The model under review builds one solid part; all positions refer to its coordinate system, in mm. Face numbers are marked on the shaded views. Give positions to 0.01 mm unless a question says otherwise; leave off trailing zeros. Order: outer loops, then holes, each group sorted by start corner. A loop starts at its lowest first (then second) coordinate and runs counter-clockwise, first axis right, second up. Notation, with made-up numbers: (82, 34.25) -> (107, 34.25) arc R12 ccw to (107, 43.25) -> close; hole circle Ø4 at (-24, 53.5). An arc over 180 degrees is marked (long way). Use one line per item in the form item = value.
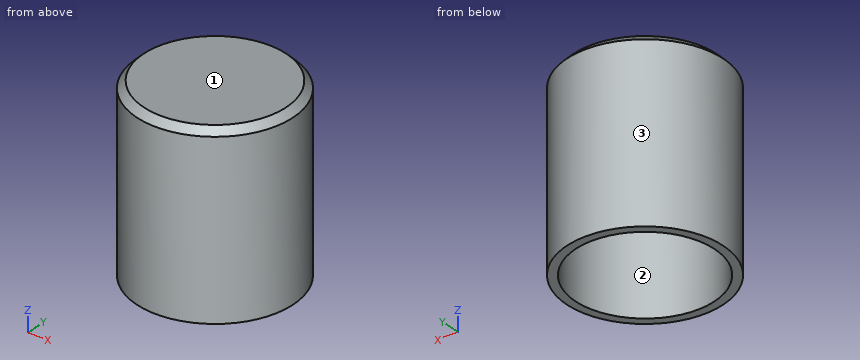
```python
from build123d import *

# Parameters (mm, degrees)
F0_R     = 22.5074090386
F1_DEPTH = 49.5
F2_DEPTH = 2
F3_SIZE  = 2
F4_T     = -2.5


with BuildPart() as f1:
    # F0 (on Top) → F1 (new body)
    with BuildSketch(Plane.XY):
        Circle(F0_R)
    extrude(amount=F1_DEPTH)

    # F2 (add): a face of the model
    f2_faces = [f1.faces().sort_by_distance(p)[0] for p in [
        (0, 0, 49.5),
    ]]
    extrude(f2_faces, amount=F2_DEPTH)

    # F3
    f3_edges = [f1.edges().sort_by_distance(p)[0] for p in [
        (-22.507409, 0, 51.5),
    ]]
    chamfer(f3_edges, length=F3_SIZE)

    # F4
    f4_openings = [f1.faces().sort_by_distance(p)[0] for p in [
        (0, 0, 0),
    ]]
    offset(amount=F4_T, openings=f4_openings)


solid = f1.part
```
1. Add section C-C on z = 32. Give the boundary of the cut face in (x, y), then the cut area to 3 significant figures.
Values:
outline = circle Ø45.01 at (0, 0); hole circle Ø40.01 at (0, 0)
area = 334 mm^2
2. Add section A-A on y = 0. Give the boundary of the cut face in (x, z).
Values:
outline = (-22.51, 0) -> (-20.01, 0) -> (-20.01, 48.46) -> (-19.47, 49) -> (19.47, 49) -> (20.01, 48.46) -> (20.01, 0) -> (22.51, 0) -> (22.51, 49.5) -> (20.51, 51.5) -> (-20.51, 51.5) -> (-22.51, 49.5) -> close
3. The part is to be moulded in two halves that separate along Y. For the marked faces 1, 2 and 3, say which applies: +Y half, -Y half, draft (parallel to the pull), parting line (faces both ways), or undercut.
Values:
face_1 = draft
face_2 = undercut
face_3 = parting line
4. For pin 1 Ø6 at (x, z) = (-14.5, 29.5) entering from +Y; pin 2 Ø10 at (x, z) = (5.5, 13.5) entering from -Y; pin 3 Ø4 at (y, z) = (-14.5, 19.5) entering from +X, all flat-tipped, find the tip position at first contact; note any pin that passes through.
Values:
pin_1 = 19.35
pin_2 = -22.5
pin_3 = 18.72
5. For L1, parallel to Y at x = 0, z = 30; L2, parallel to Z at x = -1.5, y = -12; L3, parallel to Y at x = 5, z = 43.5 (3 decimals), list the stretches that pass through material, from the lowest coordinate up.
Values:
L1 = -22.51 to -20.01, 20.01 to 22.51
L2 = 49 to 51.5
L3 = -21.945 to -19.373, 19.373 to 21.945
